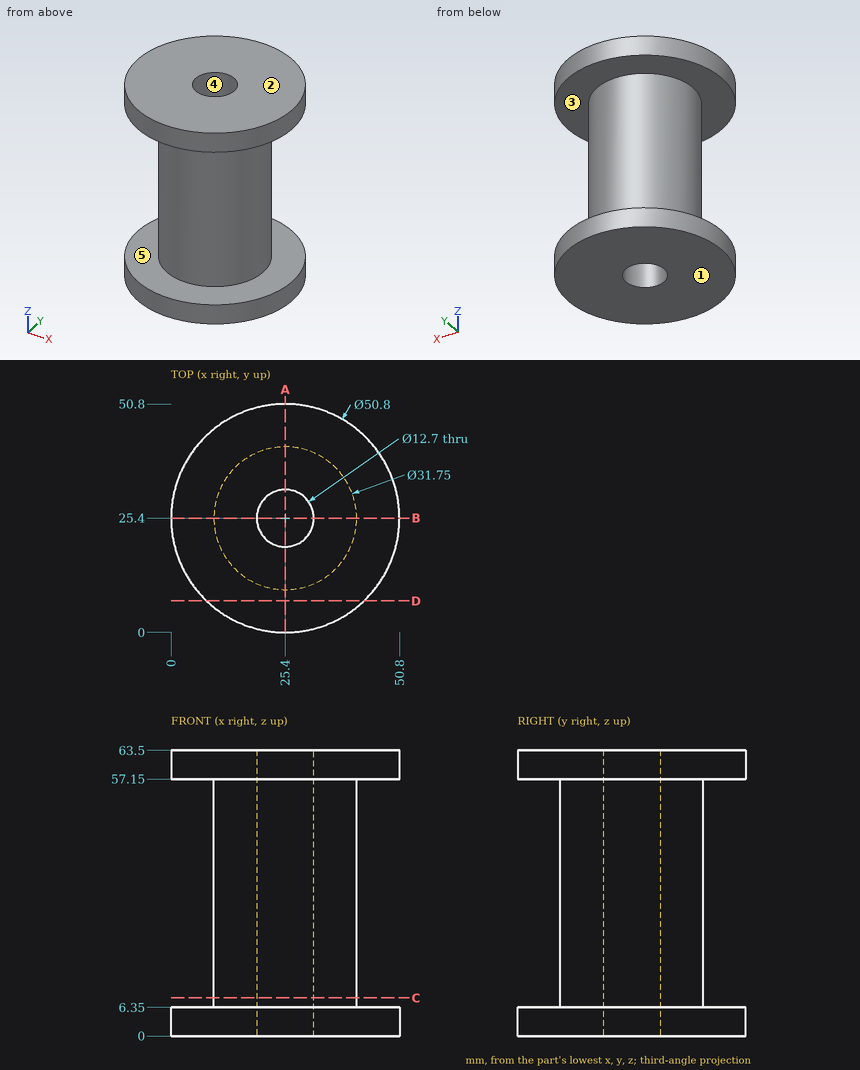
Verification items for this drawing (mm, ordinates from the low corner). A direction names the side the tool comes from. Coordinates: 2 decimals unless noted, no trailing zeros. Order: outer loops, then holes, each group sorted by start corner. A loop starts at its lowest first (then second) coordinate and runs counter-clockwise, first axis right, second up.
Q1. Sectioned sample at D-D on y = 7. Record the cut outline in (x, z), and give its area (3 significant figures).
Reply:
outline: (7.89, 0) - (42.91, 0) - (42.91, 6.35) - (7.89, 6.35) - close; (7.89, 57.15) - (42.91, 57.15) - (42.91, 63.5) - (7.89, 63.5) - close
area: 445 mm2
Q2. Draft check along Z on the marked faces 1, 2 and 3. Enter one of: released by +Z, released by -Z, zero draft, split by the parting line, or undercut.
Reply:
face 1: released by -Z
face 2: released by +Z
face 3: undercut
Q3. Sectioned sample at A-A on x = 25.4. Record the cut outline in (y, z) (3 decimals), and give its area (3 significant figures).
Reply:
outline: (0, 0) - (19.05, 0) - (19.05, 63.5) - (0, 63.5) - (0, 57.15) - (9.525, 57.15) - (9.525, 6.35) - (0, 6.35) - close; (31.75, 0) - (50.8, 0) - (50.8, 6.35) - (41.275, 6.35) - (41.275, 57.15) - (50.8, 57.15) - (50.8, 63.5) - (31.75, 63.5) - close
area: 1,450 mm2
Q4. Thickness scan on probe 1 along Z at (x, y) = (34.5, 47); probe 2 along X at (y, z) = (25, 31); probe 3 along Y at (x, z) = (25.4, 30) (3 decimals). Record the ranges inside material, lowest first.
Reply:
probe 1: z = 0 to 6.35, 57.15 to 63.5
probe 2: x = 9.53 to 19.06, 31.74 to 41.27
probe 3: y = 9.525 to 19.05, 31.75 to 41.275
Q5. Tool access check on the marked faces 4 and 5. Record the directions out of +Z, -Z, +X, -X, +Y, -Y that give a thin tool (end or side, any length) a straight path to the whole face; none if there is none.
Reply:
face 4: +Z, -Z
face 5: none
Q6. Sectioned sample at C-C on z = 8.5. Record the cut outline in (x, y) (3 decimals).
Reply:
outline: circle Ø31.75 at (25.4, 25.4); hole circle Ø12.7 at (25.4, 25.4)
Q7. Depth check by flat-ended pin: pin 1 Ø14.5 at (x, y) = (25.4, 25.4) entering from +Z; pin 2 Ø3 at (y, z) = (14, 13.5) entering from +X; pin 3 Ø2 at (x, z) = (12.5, 41.5) entering from -Y; pin 4 Ø1 at (x, z) = (20, 12) entering from -Y. Enter the tip coordinate at first touch or a pass-through.
Reply:
pin 1: stops at z = 63.5
pin 2: stops at x = 37.81
pin 3: stops at y = 14.89
pin 4: stops at y = 10.3
